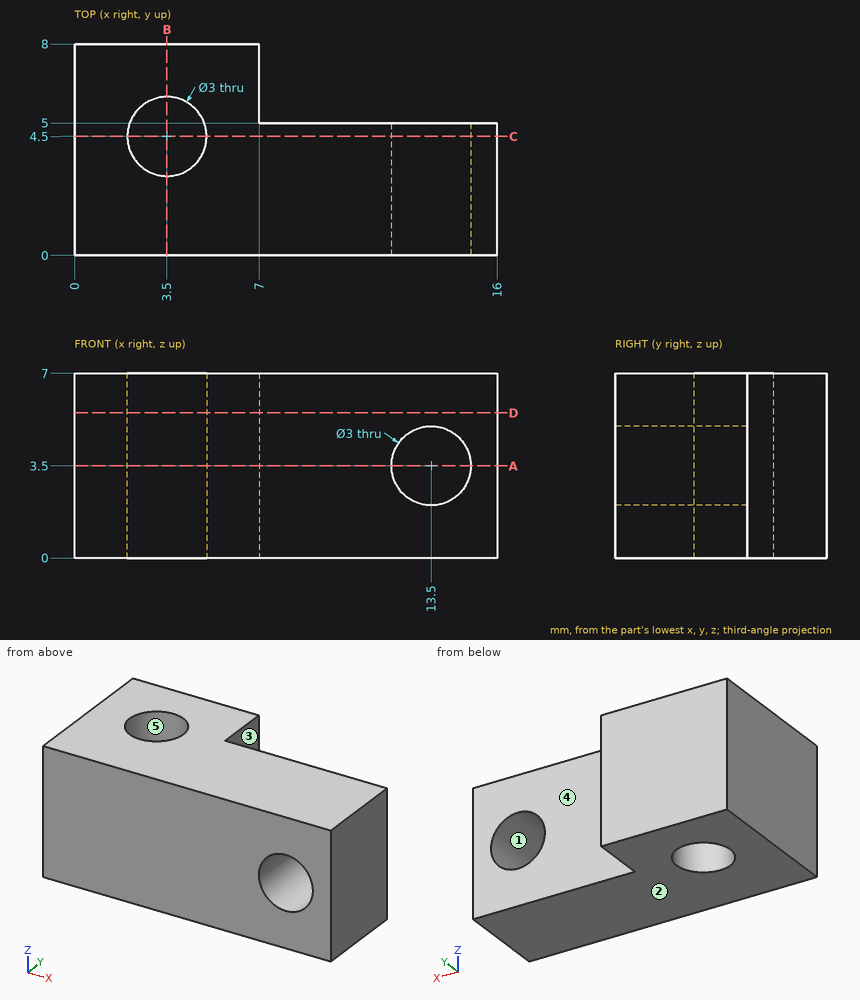
Part print with two shaded views. Sizes in mm from the minimum x, y, z corner. A direction names the side the tool comes from. Coordinates: 2 decimals unless noted, no trailing zeros. Write each loop counter-clockwise with the first axis right and the second up, starting at its lowest first coordinate (ties: lowest second). Pieces come first, ordered by that corner, then holes. Notation, with made-up numbers: M 27,12 L 81,12 A14 ccw 81,29 Z; hole C -8.5,72 d10. An arc over 180 degrees is marked long. Return JSON: item names as keys, results as strings.
Item 1: Two-plate mould, pull along Z, no slides. Class the marked faces 1, 2 and 3: +Z half, -Z half, draft (parallel to the pull), parting line (faces both ways), or undercut.
Findings below:
{"face 1": "undercut", "face 2": "-Z half", "face 3": "draft"}
Item 2: Drop flat-ended pins along their axis: pin 1 Ø1.5 at (y, z) = (6.5, 3.5) entering from +X; pin 2 Ø4 at (x, z) = (13.5, 3.5) entering from +Y. Give the stop position or say it passes through.
Findings below:
{"pin 1": "stops at x = 7", "pin 2": "stops at y = 5"}
Item 3: Slice it at D-D, the plane z = 5.5. Write the cut outline in (x, y), and give its area (3 significant figures).
Findings below:
{"outline": "M 0,0 L 16,0 L 16,5 L 7,5 L 7,8 L 0,8 Z; hole C 3.5,4.5 d3", "area": "93.9 mm2"}
Item 4: Probe line 1 (Z direction, x = 13.5, y = 1); line 2 (X direction, y = 7, z = 3); line 3 (Y direction, x = 7.25, z = 3.25). List the from-to ranges inside material, lowest first. Write a range as from..to.
Findings below:
{"line 1": "z = 0..2, 5..7", "line 2": "x = 0..7", "line 3": "y = 0..5"}
Item 5: Slice it at C-C, the plane y = 4.5. Write the cut outline in (x, z), and give its area (3 significant figures).
Findings below:
{"outline": "M 0,0 L 2,0 L 2,7 L 0,7 Z; M 5,0 L 16,0 L 16,7 L 5,7 Z; hole C 13.5,3.5 d3", "area": "83.9 mm2"}
Item 6: Slice it at B-B, the plane x = 3.5. Write the cut outline in (y, z), and give its area (3 significant figures).
Findings below:
{"outline": "M 0,0 L 3,0 L 3,7 L 0,7 Z; M 6,0 L 8,0 L 8,7 L 6,7 Z", "area": "35.0 mm2"}
Item 7: Slice it at A-A, the plane z = 3.5. Write the cut outline in (x, y).
Findings below:
{"outline": "M 0,0 L 12,0 L 12,5 L 7,5 L 7,8 L 0,8 Z; M 15,0 L 16,0 L 16,5 L 15,5 Z; hole C 3.5,4.5 d3"}
Item 8: Which spindle directions (+Z, -Z, +X, -X, +Y, -Y) get a long thin tool onto all of the face, cutting with end or side? Do the marked faces 4 and 5. Say none if no direction does.
Findings below:
{"face 4": "+Z, -Z, +X, +Y", "face 5": "+Z, -Z"}
